Design review of the part built by this model. Coordinates are the model's own, in mm. A direction names the side the tool comes from. Round coordinates to 2 decimals unless told otherwise and drop trailing zeros. Loops run counter-clockwise (first coordinate to the right, second up) from the corner with the lowest first, then second, coordinate; pieces in that order, holes last. Notation, with made-up numbers: M 55.5,-37 L 104.5,-37 A26 ccw 104.5,0 Z; hole C 58.5,25.5 d4. An arc over 180 degrees is marked long. One line per item, written item: value. Start each with the question number.
Item 1: We need section B-B (y = -6.5). Write out the cut boundary in (x, z), then the cut area to 3 significant figures.
Item 2: We need section A-A (z = 0). Write out the cut boundary in (x, y), then the cut area to 3 significant figures.
Item 3: For faces 4 (the conical face through (1.107, 1.302, 4.986)), 5 (the cylindrical face through (-5.158, -6.902, -3.955)), list the 3-axis set-ups (+Z, -Z, +X, -X, +Y, -Y) from which the entire face can be reached by the end or side of a thin tool; tool diameter is ignored.
Item 4: For line 1 along X through (y, z) = (-10, 0); line 2 along Z through (x, y) = (1.25, 0.25), list the stretches that pass through material, from the lowest coordinate up.
Item 5: Mouldability with a two-part tool opening along Z and no side actions: class faces 1 (the conical face through (1.45, 0.36, 6.51)), 2 (the flat face through (-4.42, -14, 1.54)), 3 (the cylindrical face through (-0.59, -6.9, 4.46)) as released by +Z, released by -Z, zero draft, split by the parting line, or undercut.
Item 6: Clearance check with flat-ended pins moving along their axes: pin 1 (8 mm diameter, centred on x = 1.5, y = 1.5, fed in from -Z); pin 2 (2 mm diameter, centred on x = -5.5, y = 5, fed in from -Z); pin 3 (2 mm diameter, centred on y = 3.5, z = -3.5, fed in from -X); pin 4 (2 mm diameter, centred on y = -4, z = 2.5, fed in from +X). State where each tip first meets the part, or that it passes through.
Item 7: We need section C-C (y = 5). Write out the cut boundary in (x, z), then the cut area to 3 significant figures.
from build123d import *

# Parameters (mm, degrees)
CROQUIS3_R              = 6.5
CROQUIS3_R_2            = 4.5
SALIENTE_EXTRUIR1_DEPTH = 14
CROQUIS4_W              = 14.224697916
CROQUIS4_H              = 2.830487819
CORTAR_EXTRUIR1_DEPTH   = 7.5


with BuildPart() as part:
    # Croquis2 → Revolución1 (revolve)
    with BuildSketch(Plane.XY):
        Polygon((-4.5, 0), (-8, 7.5), (-10, 7.5), (-6.5, 0), align=None)
    revolve(axis=Axis((0, 7.5, 0), (0, -1, 0)))

    # Croquis3 → Saliente-Extruir1 (add)
    with BuildSketch(Plane.XZ):
        Circle(CROQUIS3_R)
        Circle(CROQUIS3_R_2, mode=Mode.SUBTRACT)
    extrude(amount=SALIENTE_EXTRUIR1_DEPTH)

    # Croquis4 → Cortar-Extruir1 (cut)
    with BuildSketch(Plane(origin=(0, 7.5, 0), x_dir=(1, 0, 0), z_dir=(0, 1, 0))):
        with Locations((0, 9.415243909)):
            Rectangle(CROQUIS4_W, CROQUIS4_H)
    extrude(amount=-CORTAR_EXTRUIR1_DEPTH, mode=Mode.SUBTRACT)


solid = part.part
A:
1. outline: C 0,0 d13; hole C 0,0 d9
1. area: 69.1 mm2
2. outline: M -10,7.5 L -6.5,0 L -6.5,-14 L -4.5,-14 L -4.5,0 L -8,7.5 Z; M 4.5,-14 L 6.5,-14 L 6.5,0 L 10,7.5 L 8,7.5 L 4.5,0 Z
2. area: 86.0 mm2
3. face 4: +Y
3. face 5: -Y
4. line 1: -6.5 to -4.5, 4.5 to 6.5
4. line 2: -6.5 to -4.44, 4.44 to 6.5
5. face 1: split by the parting line
5. face 2: zero draft
5. face 3: undercut
6. pin 1: z = -8
6. pin 2: z = -7.81
6. pin 3: x = -8
6. pin 4: x = 6.32
7. outline: M -3.75,-8 L 3.75,-8 A8.83 ccw long Z; hole C 0,0 d13.67
7. area: 94.2 mm2
